```python
from build123d import *

# Parameters (mm, degrees)
SKETCH1_W                = 22.225
SKETCH1_H                = 76.2
BOSS_EXTRUDE1_DEPTH      = 4.7752
F_0_257_DIAMETER_HOLE1_D = 6.5278
FILLET1_R                = 0.381


with BuildPart() as part:
    # Sketch1 → Boss-Extrude1 (new body)
    with BuildSketch(Plane(origin=(0, 4.7752, 0), x_dir=(1, 0, 0), z_dir=(0, 1, 0))):
        with Locations((11.1125, -38.1)):
            Rectangle(SKETCH1_W, SKETCH1_H)
    extrude(amount=-BOSS_EXTRUDE1_DEPTH)

    # F (0.257) Diameter Hole1 (through all)
    with Locations(Plane(origin=(0, 0, 0), x_dir=(-1, 0, 0), z_dir=(0, -1, 0))):
        with Locations((-11.1125, -12.7), (-11.1125, -38.1), (-11.1125, -63.5)):
            Hole(F_0_257_DIAMETER_HOLE1_D / 2)

    # Fillet1
    fillet1_edges = [part.edges().sort_by_distance(p)[0] for p in [
        (0, 0, 38.1),
        (22.225, 0, 38.1),
        (0, 4.7752, 38.1),
        (22.225, 4.7752, 38.1),
    ]]
    fillet(fillet1_edges, radius=FILLET1_R)


solid = part.part
```
Part model, mm, in its own coordinate system. Round coordinates to 2 decimals unless told otherwise and drop trailing zeros. Loops run counter-clockwise (first coordinate to the right, second up) from the corner with the lowest first, then second, coordinate; pieces in that order, holes last.
1. Two-plate mould, pull along X, no slides. Class faces 1 (the face through (11, 2, 0)), 2 (the face through (0, 2, 39)), 3 (the face through (10.405, 2.421, 66.686)): pulls with the +X half, pulls with the -X half, needs draft (parallel to the pull), parting line crosses it, or undercut.
Solutions:
face 1: needs draft
face 2: pulls with the -X half
face 3: undercut
2. Drill centre lines: line 1 along Z through (x, y) = (8.75, 1.6); line 2 along Z through (x, y) = (12.5, 2.8); line 3 along X through (y, z) = (1.1, 38.1) (3 decimals). Where is each one in solid material? Low to high.
Solutions:
line 1: z = 0 to 10.45, 14.95 to 35.85, 40.35 to 61.25, 65.75 to 76.2
line 2: z = 0 to 9.75, 15.65 to 35.15, 41.05 to 60.55, 66.45 to 76.2
line 3: x = 0 to 7.849, 14.376 to 22.225
3. Slice it at B-B (z = 12.7). Give the cut face in (x, y) (3 decimals).
Solutions:
outline: (0, 0.381) arc R0.381 ccw to (0.381, 0) - (7.849, 0) - (7.849, 4.775) - (0.381, 4.775) arc R0.381 ccw to (0, 4.394) - close; (14.376, 0) - (21.844, 0) arc R0.381 ccw to (22.225, 0.381) - (22.225, 4.394) arc R0.381 ccw to (21.844, 4.775) - (14.376, 4.775) - close
4. Slice it at A-A (y = 3.6). Give the cut face in (x, z) (1 decimal), and give its area (3 significant figures).
Solutions:
outline: (0, 0) - (22.2, 0) - (22.2, 76.2) - (0, 76.2) - close; hole circle Ø6.5 at (11.1, 12.7); hole circle Ø6.5 at (11.1, 38.1); hole circle Ø6.5 at (11.1, 63.5)
area: 1,590 mm2
5. Flat gauge pin, fed straight in: pin 1 (8.5 mm diameter, centred on x = 11.11, z = 63.5, fed in from -Y). Where does the tip first touch, or does it go through?
Solutions:
pin 1: stops at y = 0
